Study the drawing (mm; zero at the part's minimum x, y, z) and answer. Give positions to 0.01 mm unless a question says otherwise; leave off trailing zeros. Loops run counter-clockwise (first coordinate to the right, second up) from the corner with the lowest first, then second, coordinate; pieces in that order, holes last. Notation, with made-up numbers: (14, -5.75) - (34, -5.75) arc R16 ccw to (34, 6.25) - close; hole circle Ø2 at (-28.75, 71). An arc over 180 degrees is marked (long way). Write item = value, one per line. Start each with the question number.
1) Flat-ended cylindrical pins translate along their axes: P1, Ø3, axis at x = 35.5, y = 4.5, coming from the +Z side; P2, Ø1, axis at y = 5.5, z = 79, coming from the -X side; P3, Ø1, axis at y = 3.5, z = 115, coming from the -X side; P4, Ø1, axis at x = 81.5, z = 172.5, coming from the -Y side. Find the tip coordinate at first contact, or state that the pin passes through.
2) The part is cut by section D-D on z = 194. Write down the section's boundary in (x, y), plus the area to 3 significant figures.
3) Consider probe 1 along Z at (x, y) = (35.5, 3.5); probe 2 along Z at (x, y) = (168, 0.5); probe 3 along X at (y, z) = (5.75, 90.5). Determine where each line is inside the solid, lowest interval first.
4) The part is cut by section B-B on z = 74. Write down the section's boundary in (x, y).
5) The part is cut by section A-A on x = 34. Write down the section's boundary in (y, z).
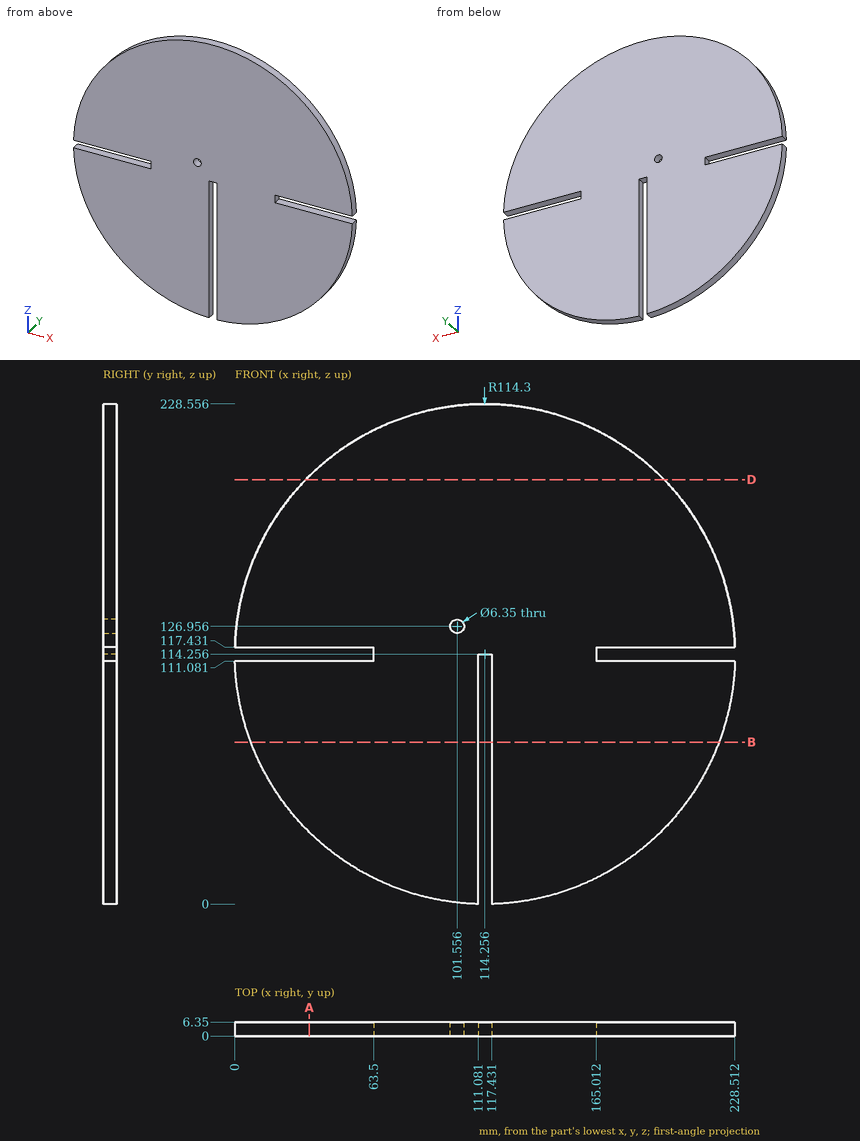
Answer below:
q1.P1 = 198.49
q1.P2 = 5.37
q1.P3 = 63.5
q1.P4 = 0
q2.outline = (32.37, 0) - (196.14, 0) - (196.14, 6.35) - (32.37, 6.35) - close
q2.area = 1,040 mm2
q3.probe_1 = 31.42 to 111.08, 117.43 to 197.09
q3.probe_2 = 13.38 to 111.08, 117.43 to 215.13
q3.probe_3 = 2.45 to 111.08, 117.43 to 226.06
q4.outline = (7.28, 0) - (111.08, 0) - (111.08, 6.35) - (7.28, 6.35) - close; (117.43, 0) - (221.23, 0) - (221.23, 6.35) - (117.43, 6.35) - close
q5.outline = (0, 32.87) - (6.35, 32.87) - (6.35, 111.08) - (0, 111.08) - close; (0, 117.43) - (6.35, 117.43) - (6.35, 195.64) - (0, 195.64) - close
